```python
from build123d import *

# Parameters (mm, degrees)
PAD040_DEPTH    = 8
PAD041_DEPTH    = 8
POCKET029_DEPTH = 14.801
POCKET030_DEPTH = 14.801
POCKET031_DEPTH = 16.001


with BuildPart() as part:
    # Sketch069 (on Face4 of Binder015) → Pad040 (new body)
    with BuildSketch(Plane.XY.offset(89.8)):
        Polygon((-86.8396103068, 95.2396103068), (-80.4396103068, 95.2396103068), (-80.4396103068, 86.8396103068), (-72.0396103068, 86.8396103068), (-72.0396103068, 80.4396103068), (-80.4396103068, 80.4396103068), (-80.4396103068, 72.0396103068), (-86.8396103068, 72.0396103068), (-86.8396103068, 80.4396103068), (-95.2396103068, 80.4396103068), (-95.2396103068, 86.8396103068), (-86.8396103068, 86.8396103068), align=None)
    extrude(amount=-PAD040_DEPTH)

    # Sketch070 (on Face13 of Pad040) → Pad041 (join)
    with BuildSketch(Plane.XY.offset(89.8)):
        Polygon((-86.8396103068, 95.2396103068), (-80.4396103068, 95.2396103068), (-80.4396103068, 86.8396103068), (-72.0396103068, 86.8396103068), (-72.0396103068, 80.4396103068), (-80.4396103068, 80.4396103068), (-80.4396103068, 72.0396103068), (-86.8396103068, 72.0396103068), (-86.8396103068, 80.4396103068), (-95.2396103068, 80.4396103068), (-95.2396103068, 86.8396103068), (-86.8396103068, 86.8396103068), align=None)
    extrude(amount=PAD041_DEPTH)

    # Sketch071 (on Face5 of Pad041) → Pocket029 (cut, through all)
    with BuildSketch(Plane(origin=(-86.8396103068, 0, 0), x_dir=(0, -1, 0), z_dir=(-1, 0, 0))):
        Polygon((-89.4325218802, 86.8), (-87.8467354426, 86.8), (-87.1396286614, 86.0928932188), (-87.1396286614, 84.5071067812), (-87.8467354426, 83.8), (-89.4325218802, 83.8), (-90.1396286614, 84.5071067812), (-90.1396286614, 86.0928932188), align=None)
        Polygon((-80.1395919522, 86.0928932188), (-80.1395919522, 84.5071067812), (-79.432485171, 83.8), (-77.8466987333, 83.8), (-77.1395919522, 84.5071067812), (-77.1395919522, 86.0928932188), (-77.8466987333, 86.8), (-79.432485171, 86.8), align=None)
        Polygon((-89.4325218802, 92.8), (-87.8467354426, 92.8), (-87.1396286614, 93.5071067812), (-87.1396286614, 95.0928932188), (-87.8467354426, 95.8), (-89.4325218802, 95.8), (-90.1396286614, 95.0928932188), (-90.1396286614, 93.5071067812), align=None)
        Polygon((-77.8466987333, 95.8), (-79.432485171, 95.8), (-80.1395919522, 95.0928932188), (-80.1395919522, 93.5071067812), (-79.432485171, 92.8), (-77.8466987333, 92.8), (-77.1395919522, 93.5071067812), (-77.1395919522, 95.0928932188), align=None)
    extrude(amount=-POCKET029_DEPTH, mode=Mode.SUBTRACT)

    # Sketch072 (on Face4 of Pocket029) → Pocket030 (cut, through all)
    with BuildSketch(Plane(origin=(0, 86.8396103068, 0), x_dir=(-1, 0, 0), z_dir=(0, 1, 0))):
        Polygon((77.8467170496, 86.8), (79.4325034872, 86.8), (80.1396102684, 86.0928932188), (80.1396102684, 84.5071067812), (79.4325034872, 83.8), (77.8467170496, 83.8), (77.1396102684, 84.5071067812), (77.1396102684, 86.0928932188), align=None)
        Polygon((87.8467171264, 86.8), (89.432503564, 86.8), (90.1396103452, 86.0928932188), (90.1396103452, 84.5071067812), (89.432503564, 83.8), (87.8467171264, 83.8), (87.1396103452, 84.5071067812), (87.1396103452, 86.0928932188), align=None)
        Polygon((77.1396102684, 95.0928932188), (77.1396102684, 93.5071067812), (77.8467170496, 92.8), (79.4325034872, 92.8), (80.1396102684, 93.5071067812), (80.1396102684, 95.0928932188), (79.4325034872, 95.8), (77.8467170496, 95.8), align=None)
        Polygon((87.1396103452, 95.0928932188), (87.1396103452, 93.5071067812), (87.8467171264, 92.8), (89.432503564, 92.8), (90.1396103452, 93.5071067812), (90.1396103452, 95.0928932188), (89.432503564, 95.8), (87.8467171264, 95.8), align=None)
    extrude(amount=-POCKET030_DEPTH, mode=Mode.SUBTRACT)

    # Sketch073 (on Face1 of Pocket030) → Pocket031 (cut, through all)
    with BuildSketch(Plane.XY.offset(97.8)):
        Polygon((-85.3396103068, 93.7396103068), (-81.9396103068, 93.7396103068), (-81.9396103068, 85.3396103068), (-73.5396103068, 85.3396103068), (-73.5396103068, 81.9396103068), (-81.9396103068, 81.9396103068), (-81.9396103068, 73.5396103068), (-85.33961, 73.53961), (-85.33961, 81.93961), (-93.73961, 81.93961), (-93.73961, 85.33961), (-85.33961, 85.33961), align=None)
    extrude(amount=-POCKET031_DEPTH, mode=Mode.SUBTRACT)


solid = part.part
```
Here's how the part is built. I have some questions about the finished solid (model axes, mm). A direction names the side the tool comes from. Coordinates: 2 decimals unless noted, no trailing zeros. Write each loop counter-clockwise with the first axis right and the second up, starting at its lowest first coordinate (ties: lowest second). Pieces come first, ordered by that corner, then holes. Notation, with made-up numbers: M -1,-13 L 38,-13 A10 ccw 38,-8 Z; hole C 27,-25.75 d9. An arc over 180 degrees is marked long. Answer as CSV lines item,"result". Start each with the question number.
Q1. Suppose I cut it at C-C, the plane y = 90.5. List the corners of the cut face in (x, z) for me.
Q2. Will these pins go through, and if not, where does the flat tip stop? pin 1 Ø1.5 at (x, z) = (-76.5, 93.5) entering from -Y; pin 2 Ø5 at (y, z) = (75.5, 91) entering from +X.
Q3. I need wall thicknesses on probe 1 along Y at (x, z) = (-93.25, 97); probe 2 along Y at (x, z) = (-85.25, 91); probe 3 along X at (y, z) = (79.25, 83.5). Which ranges of each line are inside material? Lowest first, please. Write a range as [from, to].
Q4. For faces 1 (the flat face through (-86, 87.14, 94)), 2 (the flat face through (-73.54, 84, 90)), 3 (the flat face through (-87.14, 86, 85)), which set-ups out of +Z, -Z, +X, -X, +Y, -Y let a thin tool reach every point of the face, with its end or its side?
Q5. Suppose I cut it at D-D, the plane z = 87.5. List the corners of the cut face in (x, y) for me, then the cut area to 3 significant figures.
Q6. If we mould it in two halves opening along Z, with no side actions, what happens to faces 4 (the flat face through (-90.14, 86, 94)), 5 (the flat face through (-95.24, 84, 90))? For each: pulls with the +Z half, pulls with the -Z half, needs draft (parallel to the pull), parting line crosses it, or undercut.
Q7. Suppose I cut it at A-A, the plane x = -78.75. List the corners of the cut face in (y, z) for me.
Q8. Suppose I cut it at B-B, the plane x = -93. List the corners of the cut face in (y, z) for me.
Entries:
1,outline,"M -86.84,81.8 L -85.34,81.8 L -85.34,97.8 L -86.84,97.8 Z; M -81.94,81.8 L -80.44,81.8 L -80.44,97.8 L -81.94,97.8 Z"
2,pin 1,"stops at y = 80.44"
2,pin 2,"stops at x = -80.44"
3,probe 1,"y = [80.44, 81.94], [85.34, 86.84]"
3,probe 2,"y = [72.04, 73.54], [93.74, 95.24]"
3,probe 3,"x = [-86.84, -85.34], [-81.94, -80.44]"
4,face 1,"+X, -X"
4,face 2,"+Z, -Z"
4,face 3,"+Y, -Y"
5,outline,"M -95.24,80.44 L -86.84,80.44 L -86.84,72.04 L -80.44,72.04 L -80.44,80.44 L -72.04,80.44 L -72.04,86.84 L -80.44,86.84 L -80.44,95.24 L -86.84,95.24 L -86.84,86.84 L -95.24,86.84 Z; hole M -93.74,81.94 L -85.34,81.94 L -85.34,73.54 L -81.94,73.54 L -81.94,81.94 L -73.54,81.94 L -73.54,85.34 L -81.94,85.34 L -81.94,93.74 L -85.34,93.74 L -85.34,85.34 L -93.74,85.34 Z"
5,area,"130 mm²"
6,face 4,"undercut"
6,face 5,"needs draft"
7,outline,"M 80.44,81.8 L 81.94,81.8 L 81.94,83.8 L 80.44,83.8 Z; M 80.44,86.8 L 81.94,86.8 L 81.94,92.8 L 80.44,92.8 Z; M 80.44,95.8 L 81.94,95.8 L 81.94,97.8 L 80.44,97.8 Z; M 85.34,81.8 L 86.84,81.8 L 86.84,83.8 L 85.34,83.8 Z; M 85.34,86.8 L 86.84,86.8 L 86.84,92.8 L 85.34,92.8 Z; M 85.34,95.8 L 86.84,95.8 L 86.84,97.8 L 85.34,97.8 Z"
8,outline,"M 80.44,81.8 L 81.94,81.8 L 81.94,97.8 L 80.44,97.8 Z; M 85.34,81.8 L 86.84,81.8 L 86.84,97.8 L 85.34,97.8 Z"
